```python
from build123d import *

# Parameters (mm, degrees)
BOSS_EXTRUDE1_DEPTH            = 25
SKETCH2_R                      = 2.6
CUT_EXTRUDE1_DEPTH             = 29.265728709
CUT_EXTRUDE2_REACH             = 30.266
SKETCH3_R                      = 2.6
CUT_EXTRUDE2_DIRECTION_2_DEPTH = 1
CUT_EXTRUDE3_START             = -4
SKETCH5_R                      = 5.5
CUT_EXTRUDE3_DEPTH             = 25.265728709
CUT_EXTRUDE4_START             = -4
SKETCH7_R                      = 5.5
CUT_EXTRUDE4_DEPTH             = 25.265728709


with BuildPart() as part:
    # Sketch1 → Boss-Extrude1 (new body)
    with BuildSketch(Plane.XY):
        Polygon((0, 0), (28.265728709, 28.265728709), (28.265728709, 0), align=None)
    extrude(amount=-BOSS_EXTRUDE1_DEPTH)

    # Sketch2 → Cut-Extrude1 (cut, through all)
    with BuildSketch(Plane.XZ):
        with Locations((5, -12.5)):
            Circle(SKETCH2_R)
    extrude(amount=-CUT_EXTRUDE1_DEPTH, mode=Mode.SUBTRACT)

    # Sketch3 → Cut-Extrude2 (cut, up to next)
    with BuildSketch(Plane(origin=(28.265728709, 0, 0), x_dir=(0, 0, -1), z_dir=(1, 0, 0)), mode=Mode.PRIVATE) as cut_extrude2_sk1:
        with Locations((12.5, 23.265728709)):
            Circle(SKETCH3_R)
    cut_extrude2_tool1 = extrude(cut_extrude2_sk1.sketch, amount=-CUT_EXTRUDE2_REACH, mode=Mode.PRIVATE) & part.part
    add(cut_extrude2_tool1.solids().sort_by_distance((28.265729, 23.265729, -12.5))[0], mode=Mode.SUBTRACT)

    # Sketch3 → Cut-Extrude2 direction 2 (cut)
    with BuildSketch(Plane(origin=(28.265728709, 0, 0), x_dir=(0, 0, -1), z_dir=(1, 0, 0))):
        with Locations((12.5, 23.265728709)):
            Circle(SKETCH3_R)
    extrude(amount=CUT_EXTRUDE2_DIRECTION_2_DEPTH, mode=Mode.SUBTRACT)

    # Sketch5 → Cut-Extrude3 (cut, through all)
    with BuildSketch(Plane(origin=(28.265728709, 0, 0), x_dir=(0, 0, -1), z_dir=(1, 0, 0)).offset(CUT_EXTRUDE3_START)):
        with Locations((12.5, 23.265728709)):
            Circle(SKETCH5_R)
    extrude(amount=-CUT_EXTRUDE3_DEPTH, mode=Mode.SUBTRACT)

    # Sketch7 → Cut-Extrude4 (cut, through all)
    with BuildSketch(Plane.XZ.offset(CUT_EXTRUDE4_START)):
        with Locations((5, -12.5)):
            Circle(SKETCH7_R)
    extrude(amount=-CUT_EXTRUDE4_DEPTH, mode=Mode.SUBTRACT)


solid = part.part
```
For this review, take the finished solid that the model builds, in its own axes (mm). Round coordinates to 2 decimals unless told otherwise and drop trailing zeros. Write each loop counter-clockwise with the first axis right and the second up, starting at its lowest first coordinate (ties: lowest second). Pieces come first, ordered by that corner, then holes. Notation, with made-up numbers: (-24, 73.5) - (-13, 73.5) arc R19 cw to (-13, 92.5) - close; hole circle Ø11 at (5.25, -6). An arc over 180 degrees is marked (long way). Answer as CSV lines item,"result". Start each with the question number.
(1) Mouldability with a two-part tool opening along X and no side actions: class faces 1 (the flat face through (24.266, 20, -12)), 2 (the cylindrical face through (7.4, 2, -13.5)), 3 (the flat face through (28.266, 14, -12)), 4 (the flat face through (21, 8, -25)) as +X half, -X half, draft (parallel to the pull), parting line (faces both ways), or undercut.
(2) For line 1 (Z direction, x = 5, y = 1.9); line 2 (Y direction, x = 7, z = -10.25); line 3 (Y direction, x = 10.5, z = -13.5), list the stretches that pass through material, from the lowest coordinate up.
(3) Add section D-D, the plane x = 17.25. State the section outline as (y, z) points.
(4) For pin 1 (1.5 mm diameter, centred on y = 6, z = -20, fed in from -X); pin 2 (9 mm diameter, centred on y = 23.27, z = -12.5, fed in from -X); pin 3 (8.5 mm diameter, centred on x = 5, z = -12.5, fed in from +Y), all flat-tipped, find the tip position at first contact; note any pin that passes through.
(5) Add section C-C, the plane y = 19.75. State the section outline as (x, z) points, plus the area to 3 significant figures.
(6) Add section A-A, the plane z = -12.5. State the section outline as (x, y) points.
(7) Add section B-B, the plane x = 5.25. State the section outline as (y, z) points, plus the area to 3 significant figures.
From the geometry:
1,face 1,"-X half"
1,face 2,"undercut"
1,face 3,"+X half"
1,face 4,"draft"
2,line 1,"z = -25 to -15.1, -9.9 to 0"
2,line 2,"y = 0 to 4"
2,line 3,"y = 0 to 10.5"
3,outline,"(0, -25) - (17.25, -25) - (17.25, 0) - (0, 0) - close"
4,pin 1,"stops at x = 5.25"
4,pin 2,"stops at x = 24.27"
4,pin 3,"stops at y = 4"
5,outline,"(19.75, -25) - (28.27, -25) - (28.27, 0) - (19.75, 0) - (19.75, -8.27) - (24.27, -8.27) - (24.27, -16.73) - (19.75, -16.73) - close"
5,area,"175 mm²"
6,outline,"(0, 0) - (2.4, 0) - (2.4, 2.4) - close; (7.6, 0) - (28.27, 0) - (28.27, 20.67) - (24.27, 20.67) - (24.27, 17.77) - (17.77, 17.77) - (10.5, 10.5) - (10.5, 4) - (7.6, 4) - close; (25.87, 25.87) - (28.27, 25.87) - (28.27, 28.27) - close"
7,outline,"(0, -25) - (5.25, -25) - (5.25, -17.99) - (4, -17.99) - (4, -15.09) - (0, -15.09) - close; (0, -9.91) - (4, -9.91) - (4, -7.01) - (5.25, -7.01) - (5.25, 0) - (0, 0) - close"
7,area,"96.8 mm²"
